Input: part model. Units: mm. Frame: model coordinates. Coordinates: 2 decimals unless noted, no trailing zeros. Write each loop counter-clockwise with the first axis right and the second up, starting at its lowest first coordinate (ties: lowest second). Pieces come first, ordered by that corner, then holes. Notation, with made-up numbers: (13.5, 15) - (26.5, 15) arc R19 cw to (26.5, 29) - close; hole circle Ø7 at (66, 33.25). An arc over 180 degrees is marked (long way). Put each result on its own line as item: value. Start each with the question number.
1. Cut plane A-A, the plane z = 127.5. Return loops of the section in (x, y).
2. Line query: line 1 (Z direction, x = 0, y = -10.9); line 2 (Y direction, x = 6.25, z = 277.5). Output: solid intervals per line, ascending.
3. Pin query (flat end, axial travel): pin 1 (8 mm diameter, centred on x = 0, z = 406.4, fed in from -Y); pin 2 (4 mm diameter, centred on x = -5.5, y = -8, fed in from -Z). Return the tip coordinate at first contact, or that it passes through.
from build123d import *

# Parameters (mm, degrees)
SKETCH1_W           = 25.4
SKETCH1_H           = 25.4
SKETCH1_W_2         = 20.32
SKETCH1_H_2         = 20.32
EXTRUDE_THIN1_DEPTH = 412.75
SKETCH2_R           = 2.4892
CUT_EXTRUDE1_DEPTH  = 26.4
SKETCH3_R           = 3.175
CUT_EXTRUDE2_DEPTH  = 26.4


with BuildPart() as part:
    # Sketch1 → Extrude-Thin1 (new body)
    with BuildSketch(Plane.XY):
        Rectangle(SKETCH1_W, SKETCH1_H)
        Rectangle(SKETCH1_W_2, SKETCH1_H_2, mode=Mode.SUBTRACT)
    extrude(amount=EXTRUDE_THIN1_DEPTH)

    # Sketch2 → Cut-Extrude1 (cut, through all)
    with BuildSketch(Plane(origin=(0, 12.7, 0), x_dir=(1, 0, 0), z_dir=(0, 1, 0))):
        with Locations((0, -406.4)):
            Circle(SKETCH2_R)
        with Locations((0, -368.3)):
            Circle(SKETCH2_R)
    extrude(amount=-CUT_EXTRUDE1_DEPTH, mode=Mode.SUBTRACT)

    # Sketch3 → Cut-Extrude2 (cut, through all)
    with BuildSketch(Plane(origin=(12.7, 0, 0), x_dir=(0, 0, -1), z_dir=(1, 0, 0))):
        with Locations((-6.35, 0)):
            Circle(SKETCH3_R)
    extrude(amount=-CUT_EXTRUDE2_DEPTH, mode=Mode.SUBTRACT)


solid = part.part
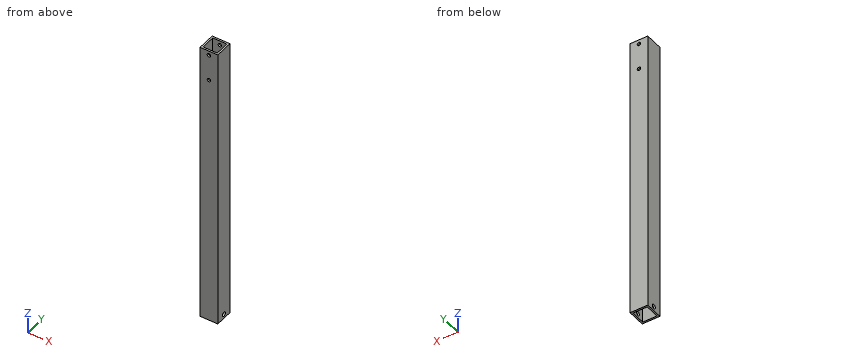
Report:
1. outline: (-12.7, -12.7) - (12.7, -12.7) - (12.7, 12.7) - (-12.7, 12.7) - close; hole (-10.16, -10.16) - (10.16, -10.16) - (10.16, 10.16) - (-10.16, 10.16) - close
2. line 1: z = 0 to 365.81, 370.79 to 403.91, 408.89 to 412.75
2. line 2: y = -12.7 to -10.16, 10.16 to 12.7
3. pin 1: stops at y = -12.7
3. pin 2: passes through
